Check sheet for the modelled part. Datum: model origin and axes. Units: mm. Give positions to 0.01 mm unless a question says otherwise; leave off trailing zeros. Loops run counter-clockwise (first coordinate to the right, second up) from the corner with the lowest first, then second, coordinate; pieces in that order, holes last. Notation, with made-up numbers: (21.25, 60.25) -> (75.25, 60.25) arc R23 cw to (75.25, 71.25) -> close; hole circle Ø10 at (89.25, 24.25). An arc over 180 degrees is marked (long way). Write each question's results on one line, items separated by ' | '. Start each with the question number.
Item 1: Scan lines: line 1 along X through (y, z) = (10, -13); line 2 along Z through (x, y) = (16, 11); line 3 along Z through (x, y) = (-17, -54). Record each from-to range of solid material in increasing order.
Item 2: Gauge pin test, flat ends, axial feed: pin 1 Ø2 at (y, z) = (-40.5, -36.5) entering from -X; pin 2 Ø1 at (x, y) = (-34.5, -46) entering from +Z; pin 3 Ø10 at (y, z) = (51, -26) entering from +X. Record the tip position at first contact, or that the pin passes through.
Item 3: Cross-section at B-B on z = -25.5. Enter the section's corners in (x, y), then the cut area to 3 significant figures.
Item 4: Cross-section at C-C on x = -18. Enter the section's corners in (y, z).
Item 5: Cross-section at A-A on y = -9. Enter the section's corners in (x, z).
from build123d import *

# Parameters (mm, degrees)
F1_DEPTH = 100


with BuildPart() as f1:
    # F0 (on Front) → F1 (new body, symmetric)
    with BuildSketch(Plane.XZ):
        Polygon((-15.199252, 48.053728), (-38.766231, 32.208033), (-50.025206, 6.136514), (-45.401532, -21.883304), (-26.363192, -42.955328), (1.045276, -50.389339), (28.121875, -41.825091), (46.269978, -19.981672), (49.72769, 8.205787), (37.397212, 33.787966), (13.193383, 48.642705), align=None)
    extrude(amount=F1_DEPTH, both=True)


solid = f1.part
Answer sheet:
1) line 1: x = -46.87 to 47.13 | line 2: z = -45.66 to 46.92 | line 3: z = -45.49 to 46.84
2) pin 1: stops at x = -33.1 | pin 2: stops at z = 35.41 | pin 3: stops at x = 45.42
3) outline: (-42.13, -100) -> (41.69, -100) -> (41.69, 100) -> (-42.13, 100) -> close | area: 16,800 mm²
4) outline: (-100, -45.22) -> (100, -45.22) -> (100, 46.17) -> (-100, 46.17) -> close
5) outline: (-50.03, 6.14) -> (-45.4, -21.88) -> (-26.36, -42.96) -> (1.05, -50.39) -> (28.12, -41.83) -> (46.27, -19.98) -> (49.73, 8.21) -> (37.4, 33.79) -> (13.19, 48.64) -> (-15.2, 48.05) -> (-38.77, 32.21) -> close
